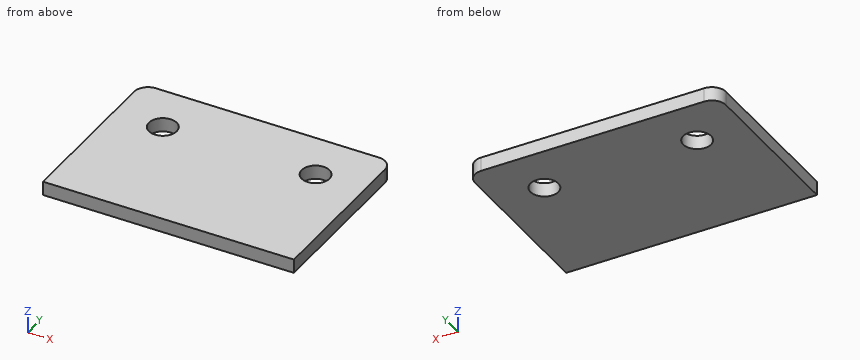
```python
from build123d import *

# Parameters (mm, degrees)
BOSS_EXTRUDE1_DEPTH = 3.175
SKETCH2_R           = 3.175
CUT_EXTRUDE1_DEPTH  = 67.929307933
SKETCH3_W           = 57.15
SKETCH3_H           = 29.175717927
CUT_EXTRUDE2_DEPTH  = 5.08


with BuildPart() as part:
    # Sketch1 → Boss-Extrude1 (new body)
    with BuildSketch(Plane.XY):
        with BuildLine():
            Line((-28.328951223, 3.070773738), (-28.328951223, -34.922456704))
            Line((-28.328951223, -34.922456704), (-28.328951223, -57.147456704))
            ThreePointArc((-28.328951223, -57.147456704), (-27.399015253, -59.392520734), (-25.153951223, -60.322456704))
            Line((-25.153951223, -60.322456704), (25.646048777, -60.322456704))
            ThreePointArc((25.646048777, -60.322456704), (27.891112807, -59.392520734), (28.821048777, -57.147456704))
            Line((28.821048777, -57.147456704), (28.821048777, -34.922456704))
            Line((28.821048777, -34.922456704), (28.821048777, 3.070773738))
            ThreePointArc((28.821048777, 3.070773738), (27.891112807, 5.315837768), (25.646048777, 6.245773738))
            Line((25.646048777, 6.245773738), (-25.153951223, 6.245773738))
            ThreePointArc((-25.153951223, 6.245773738), (-27.399015253, 5.315837768), (-28.328951223, 3.070773738))
        make_face()
    extrude(amount=-BOSS_EXTRUDE1_DEPTH)

    # Sketch2 → Cut-Extrude1 (cut, through all)
    with BuildSketch(Plane.XY):
        with Locations((-17.152951223, -5.184226262)):
            Circle(SKETCH2_R)
        with Locations(Location((17.645048777, -5.184226262, 0), (0, 0, 180))):
            Circle(SKETCH2_R)
    extrude(amount=-CUT_EXTRUDE1_DEPTH, mode=Mode.SUBTRACT)

    # Sketch3 → Cut-Extrude2 (cut)
    with BuildSketch(Plane(origin=(0, 0, -3.175), x_dir=(-1, 0, 0), z_dir=(0, 0, -1))):
        with Locations((-0.246048777, -48.534555274)):
            Rectangle(SKETCH3_W, SKETCH3_H)
    extrude(amount=-CUT_EXTRUDE2_DEPTH, mode=Mode.SUBTRACT)


solid = part.part
```
The model under review builds one solid part; all positions refer to its coordinate system, in mm. Give positions to 0.01 mm unless a question says otherwise; leave off trailing zeros. Write each loop counter-clockwise with the first axis right and the second up, starting at its lowest first coordinate (ties: lowest second). Pieces come first, ordered by that corner, then holes.
(1) For P1, Ø5.5, axis at x = 17.65, y = -5.18, coming from the -Z side, flat-tipped, find the tip position at first contact; note if it passes through.
(2) To check wall thickness, follow L1, parallel to X at y = -6, z = -1.85; L2, parallel to X at y = -5.5, z = -0.45; L3, parallel to Y at x = 18.5, z = -1.05. State the ranges of each line that lie inside material, in increasing order.
(3) Consider section B-B, the plane x = 20. Give the boundary of the cut face in (y, z) (3 decimals).
(4) Consider section A-A, the plane z = -1.1. Give the boundary of the cut face in (x, y) (3 decimals), and give its area (3 significant figures).
(5) Consider section C-C, the plane x = -19.5. Give the boundary of the cut face in (y, z) (3 decimals), and give its area (3 significant figures).
Returned:
1. P1: passes through
2. L1: x = -28.33 to -20.22, -14.08 to 14.58, 20.71 to 28.82
2. L2: x = -28.33 to -20.31, -13.99 to 14.49, 20.8 to 28.82
2. L3: y = -33.95 to -8.24, -2.13 to 6.25
3. outline: (-33.947, -3.175) - (-7.314, -3.175) - (-7.314, 0) - (-33.947, 0) - close; (-3.055, -3.175) - (6.246, -3.175) - (6.246, 0) - (-3.055, 0) - close
4. outline: (-28.329, -33.947) - (28.821, -33.947) - (28.821, 3.071) arc R3.175 ccw to (25.646, 6.246) - (-25.154, 6.246) arc R3.175 ccw to (-28.329, 3.071) - close; hole circle Ø6.35 at (-17.153, -5.184); hole circle Ø6.35 at (17.645, -5.184)
4. area: 2,230 mm2
5. outline: (-33.947, -3.175) - (-7.322, -3.175) - (-7.322, 0) - (-33.947, 0) - close; (-3.046, -3.175) - (6.246, -3.175) - (6.246, 0) - (-3.046, 0) - close
5. area: 114 mm2
